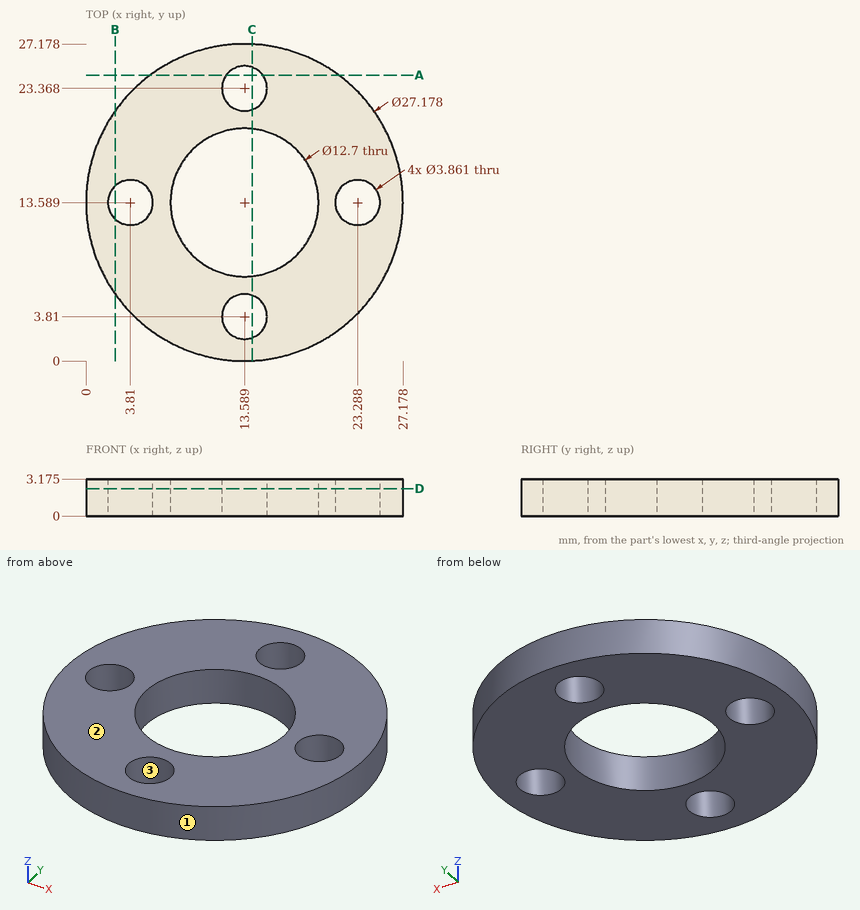
Drawing for the job (mm, zero at the part's lowest x, y, z). Give positions to 0.01 mm unless a question says otherwise; leave off trailing zeros. Order: outer loops, then holes, each group sorted by start corner. A loop starts at its lowest first (then second) coordinate and runs counter-clockwise, first axis right, second up. Notation, with made-up numbers: (3, 79) - (23, 79) arc R18 ccw to (23, 84) - close; hole circle Ø11 at (-35.5, 19). An arc over 180 degrees is marked (long way). Write item = value, one per line. Start each with the question number.
1. Cut at A-A, the plane y = 24.5. List the corners of the cut face in (x, z) (1 decimal), and give its area (3 significant figures).
2. Probe line 1 along Y through (x, z) = (12.5, 1.7) (1 decimal); line 2 along Y through (x, z) = (5.5, 1.8) (1 decimal); line 3 along Y through (x, z) = (24.5, 2.95) (1 decimal). List the from-to ranges inside material, lowest first.
3. Cut at B-B, the plane x = 2.5. List the corners of the cut face in (y, z) (1 decimal), and give its area (3 significant figures).
4. Cut at C-C, the plane x = 14.25. List the corners of the cut face in (y, z) (1 decimal).
5. Two-plate mould, pull along X, no slides. Class the marked faces 1, 2 and 3: pulls with the +X half, pulls with the -X half, needs draft (parallel to the pull), parting line crosses it, or undercut.
6. Drop flat-ended pins along their axis: P1, Ø8, axis at x = 11.5, y = 13, coming from the +Z side; P2, Ø1, axis at x = 11.5, z = 2, coming from the +Y side (1 decimal). Give the stop position or say it passes through.
7. Cut at D-D, the plane z = 2.35. List the corners of the cut face in (x, y), and give its area (3 significant figures).
Taken from the geometry:
q1.outline = (5.5, 0) - (12, 0) - (12, 3.2) - (5.5, 3.2) - close; (15.2, 0) - (21.7, 0) - (21.7, 3.2) - (15.2, 3.2) - close
q1.area = 41.5 mm²
q2.line_1 = 0 to 2.2, 5.4 to 7.3, 19.8 to 21.8, 25 to 27.1
q2.line_2 = 2.7 to 12.7, 14.5 to 24.5
q2.line_3 = 5.5 to 12.1, 15.1 to 21.7
q3.outline = (5.7, 0) - (12.2, 0) - (12.2, 3.2) - (5.7, 3.2) - close; (15, 0) - (21.4, 0) - (21.4, 3.2) - (15, 3.2) - close
q3.area = 40.9 mm²
q4.outline = (0, 0) - (2, 0) - (2, 3.2) - (0, 3.2) - close; (5.6, 0) - (7.3, 0) - (7.3, 3.2) - (5.6, 3.2) - close; (19.9, 0) - (21.6, 0) - (21.6, 3.2) - (19.9, 3.2) - close; (25.2, 0) - (27.2, 0) - (27.2, 3.2) - (25.2, 3.2) - close
q5.face_1 = parting line crosses it
q5.face_2 = needs draft
q5.face_3 = undercut
q6.P1 = through
q6.P2 = 27.1
q7.outline = circle Ø27.18 at (13.59, 13.59); hole circle Ø3.86 at (3.81, 13.59); hole circle Ø12.7 at (13.59, 13.59); hole circle Ø3.86 at (13.59, 3.81); hole circle Ø3.86 at (13.59, 23.37); hole circle Ø3.86 at (23.29, 13.59)
q7.area = 407 mm²
